Work out the finished part from the listing and answer in its coordinate system (mm). Face numbers are marked on the shaded views. A direction names the side the tool comes from. Round coordinates to 2 decimals unless told otherwise and drop trailing zeros. Loops run counter-clockwise (first coordinate to the right, second up) from the corner with the lowest first, then second, coordinate; pieces in that order, holes last. Notation, with made-up numbers: (-1, 63.5) -> (16, 63.5) arc R20 ccw to (16, 81.5) -> close; hole circle Ø4 at (47, 14). An arc over 180 degrees is marked (long way). Use one line per item in the form item = value.
Autodesk Inventor part; units mm, degrees
ref_plane "YZ Plane" through (0, 0, 0) normal (1, 0, 0) x (0, 1, 0)
ref_plane "XZ Plane" through (0, 0, 0) normal (0, 1, 0) x (-1, 0, 0)
ref_plane "XY Plane" through (0, 0, 0) normal (0, 0, 1) x (1, 0, 0)
sketch "Sketch1" plane through (0, 0, 0) normal (0, 0, 1) x (1, 0, 0)
  circle A0 centre (0, 0) radius 1.7145
  circle A1 centre (0, 41.91) radius 1.7145
  arc A2 (0, 38.4175) -> (-2.4156, 44.4323) centre (0, 41.91) ccw
  arc A3 (-2.4156, -2.5223) -> (0, 3.4925) centre (0, 0) ccw
  line L0 (0, 3.4925) -> (-3.175, 3.4925)
  line L1 (-3.175, 3.4925) -> (-3.175, 38.4175)
  line L2 (-3.175, 38.4175) -> (0, 38.4175)
  line L3 (-9.525, 37.6238) -> (-9.525, 4.2862)
  line L4 (-9.525, 4.2862) -> (-2.4156, -2.5223)
  line L5 (-9.525, 37.6238) -> (-2.4156, 44.4323)
  dimension "d0" = 3.429
  dimension "d1" = 3.429
  dimension "d2" = 6.985
  dimension "d3" = 6.985
  dimension "d4" = 3.175
  dimension "d5" = 41.91
  dimension "d6" = 33.3375
  dimension "d13" = 9.525
extrude "Extrusion1" add sketch "Sketch1" along normal blind 4.7625
sketch "Sketch2" plane through (-9.525, 4.2862, 0) normal (-1, 0, 0) x (0, 0, 1)
  circle A0 centre (2.3812, 30.9563) radius 1.0795
  circle A1 centre (2.3812, 2.3813) radius 1.0795
  line L0 (0, 33.3375) -> (4.7625, 33.3375) construction
  line L1 (2.3812, 30.9563) -> (2.3812, 2.3813) construction
  line L2 (0, 0) -> (0, 33.3375) construction
  point P0 (0, -4.2862)
  point P1 (2.3813, 33.3375)
  point P2 (2.3813, 16.6688)
  point P3 (0, 16.6688)
  dimension "d9" = 28.575
  dimension "d10" = 2.159
extrude "Extrusion2" cut sketch "Sketch2" against normal through all
sketch "Sketch3" plane through (-9.525, 4.2862, 0) normal (-1, 0, 0) x (0, 0, 1)
  circle A0 centre (2.3812, 30.9563) radius 1.0795 construction
  circle A1 centre (2.3812, 2.3813) radius 1.0795 construction
  line L0 (0, 0) -> (0, 33.3375) construction
  line L1 (0, 0) -> (4.7625, 0) construction
  line L2 (4.7625, 33.3375) -> (4.7625, 0) construction
  line L3 (0, 33.3375) -> (4.7625, 33.3375) construction
  line L4 (4.7625, -0.7937) -> (4.7625, 34.1313)
  line L5 (0, 28.4163) -> (4.7625, 28.4163)
  line L6 (4.7625, 28.4163) -> (4.7625, 4.9212)
  line L7 (4.7625, 4.9212) -> (0, 4.9212)
  line L8 (0, 4.9212) -> (0, 28.4163)
  point P0 (0, -4.2862)
  point P1 (4.7625, 16.6688)
  point P2 (4.7625, 16.6688)
  dimension "d14" = 23.495
extrude "Extrusion3" cut sketch "Sketch3" against normal blind 3.175
properties part number "relayHolder2" material "ABS Plastic"
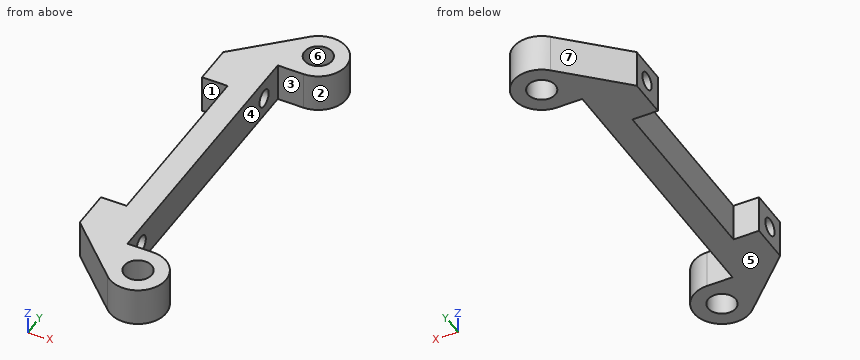
(1) Find section C-C, the plane y = 0. Write down the section's boundary in (x, z).
Completed:
outline = (-5.05, 0) -> (-1.71, 0) -> (-1.71, 4.76) -> (-5.05, 4.76) -> close; (1.71, 0) -> (3.49, 0) -> (3.49, 4.76) -> (1.71, 4.76) -> close
(2) Find section B-B, the plane z = 4.35. State how many separate pieces and enclosed holes the cut face has, then the cut area to 3 significant figures.
Completed:
separate_pieces = 1
enclosed_holes = 2
area = 236 mm2
(3) Find section A-A, the plane x = -7. Write down the section's boundary in (y, z).
Completed:
outline = (1.87, 0) -> (9.21, 0) -> (9.21, 4.76) -> (1.87, 4.76) -> close; (32.7, 0) -> (40.04, 0) -> (40.04, 4.76) -> (32.7, 4.76) -> close; hole circle Ø2.16 at (6.67, 2.38); hole circle Ø2.16 at (35.24, 2.38)
(4) Find section D-D, the plane x = 2.5. Write down the section's boundary in (y, z), then the cut area to 3 significant figures.
Completed:
outline = (-2.44, 0) -> (2.44, 0) -> (2.44, 4.76) -> (-2.44, 4.76) -> close; (39.47, 0) -> (44.35, 0) -> (44.35, 4.76) -> (39.47, 4.76) -> close
area = 46.5 mm2
(5) Consider L1, parallel to Y at x = 0, z = 1.6; L2, parallel to Y at x = -7.75, z = 1.85; L3, parallel to X at y = 8, z = 2.5 (3 decimals). Determine where each line is inside the solid, lowest interval first.
Completed:
L1 = -3.49 to -1.71, 1.71 to 3.49, 38.42 to 40.2, 43.62 to 45.4
L2 = 2.59 to 5.73, 7.61 to 9.21, 32.7 to 34.3, 36.18 to 39.32
L3 = -9.525 to -3.175
(6) For the marked faces 1, 2 and 3, determine the directions among +Z, -Z, +X, -X, +Y, -Y from which every point of the face is accessible in a straight line to the end or side of a thin tool.
Completed:
face_1 = +Z, -Z, -X
face_2 = +Z, -Z
face_3 = +Z, -Z, +X
(7) For a pull along Y with two mould halves and no side action, classify the marked faces 4, 5, 6 and 7 as +Y half, -Y half, draft (parallel to the pull), parting line (faces both ways), or undercut.
Completed:
face_4 = undercut
face_5 = draft
face_6 = undercut
face_7 = +Y half
(8) Given P1, Ø2.5, axis at x = -7, z = 2, coming from the +Y side; P2, Ø2.5, axis at x = -1.5, z = 1.5, coming from the +Y side; P3, Ø2.5, axis at x = -8.5, z = 2, coming from the -Y side, each flat-ended and moving along its own axis, determine where each tip first touches the part or whether it passes through.
Completed:
P1 = 41.24
P2 = 45.39
P3 = 2.11
